Read the model definition and answer for the solid it produces. Units are mm, in the model's axes. Coordinates: 2 decimals unless noted, no trailing zeros. Order: outer loops, then holes, each group sorted by start corner. A loop starts at its lowest first (then second) coordinate and runs counter-clockwise, first axis right, second up.
```python
from build123d import *

# Parameters (mm, degrees)
SKETCH1_W           = 500
SKETCH1_H           = 500
BOSS_EXTRUDE1_DEPTH = 6.35
SKETCH2_R           = 84
CUT_EXTRUDE1_DEPTH  = 6.35
CUT_EXTRUDE3_DEPTH  = 6.35
FILLET1_R           = 15


with BuildPart() as part:
    # Sketch1 → Boss-Extrude1 (new body)
    with BuildSketch(Plane(origin=(0, 0, 0), x_dir=(1, 0, 0), z_dir=(0, 1, 0))):
        with Locations((48.037604912, -85.456276451)):
            Rectangle(SKETCH1_W, SKETCH1_H)
    extrude(amount=BOSS_EXTRUDE1_DEPTH)

    # Sketch2 → Cut-Extrude1 (cut)
    with BuildSketch(Plane(origin=(0, 6.35, 0), x_dir=(1, 0, 0), z_dir=(0, 1, 0))):
        with Locations((48.037604912, -85.456276451)):
            Circle(SKETCH2_R)
    extrude(amount=-CUT_EXTRUDE1_DEPTH, mode=Mode.SUBTRACT)

    # Sketch3 → Cut-Extrude3 (cut)
    with BuildSketch(Plane(origin=(0, 6.35, 0), x_dir=(1, 0, 0), z_dir=(0, 1, 0))):
        Polygon((216.329018834, 78.592496784), (103.191933845, -34.544588206), (98.949293158, -30.301947519), (212.086378147, 82.835137471), align=None)
        Polygon((-120.25380901, 78.592496784), (-116.011168323, 82.835137471), (-2.874083333, -30.301947519), (-7.11672402, -34.544588206), align=None)
        Polygon((212.086378147, -253.747690374), (98.949293158, -140.610605384), (103.191933845, -136.367964697), (216.329018835, -249.505049687), align=None)
        Polygon((-120.25380901, -249.505049687), (-7.11672402, -136.367964697), (-2.874083333, -140.610605384), (-116.011168323, -253.747690374), align=None)
    extrude(amount=-CUT_EXTRUDE3_DEPTH, mode=Mode.SUBTRACT)

    # Fillet1
    fillet1_edges = [part.edges().sort_by_distance(p)[0] for p in [
        (105.275361381, 3.175, 23.975879296),
        (109.518002068, 3.175, 28.218519983),
        (109.518002068, 3.175, 142.69403292),
        (105.275361381, 3.175, 146.936673607),
        (-13.442792244, 3.175, 142.69403292),
        (-9.200151557, 3.175, 146.936673607),
        (-13.442792244, 3.175, 28.218519983),
        (-9.200151557, 3.175, 23.975879296),
    ]]
    fillet(fillet1_edges, radius=FILLET1_R)


solid = part.part
```
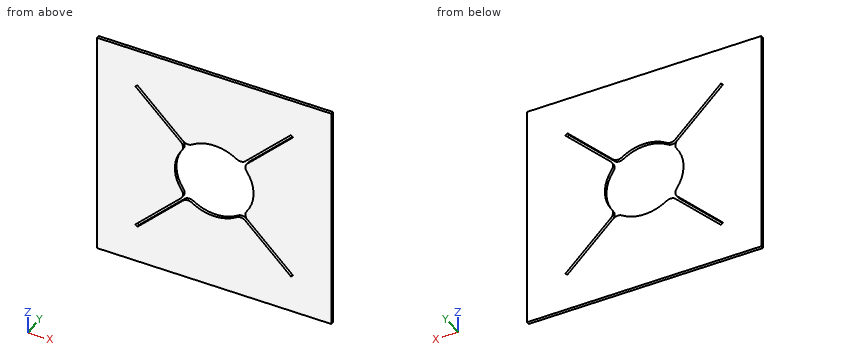
1) A cutting plane is placed at B-B, the plane y = 4.5. Determine the outline of the cut face in (x, z), and give its area (3 significant figures).
A:
outline: (-201.96, -164.54) - (298.04, -164.54) - (298.04, 335.46) - (-201.96, 335.46) - close; hole (-120.25, -78.59) - (-116.01, -82.84) - (-18.68, 14.5) arc R15 cw to (0.43, 16.25) arc R84 ccw to (95.65, 16.25) arc R15 cw to (114.75, 14.5) - (212.09, -82.84) - (216.33, -78.59) - (119, 18.74) arc R15 cw to (117.24, 37.85) arc R84 ccw to (117.24, 133.06) arc R15 cw to (119, 152.17) - (216.33, 249.51) - (212.09, 253.75) - (114.75, 156.41) arc R15 cw to (95.65, 154.66) arc R84 ccw to (0.43, 154.66) arc R15 cw to (-18.68, 156.41) - (-116.01, 253.75) - (-120.25, 249.51) - (-22.92, 152.17) arc R15 cw to (-21.17, 133.06) arc R84 ccw to (-21.17, 37.85) arc R15 cw to (-22.92, 18.74) - close
area: 224,000 mm2
2) A cutting plane is placed at A-A, the plane x = -87. Determine the outline of the cut face in (y, z).
A:
outline: (0, -164.54) - (6.35, -164.54) - (6.35, -53.82) - (0, -53.82) - close; (0, -45.34) - (6.35, -45.34) - (6.35, 216.25) - (0, 216.25) - close; (0, 224.74) - (6.35, 224.74) - (6.35, 335.46) - (0, 335.46) - close
3) A cutting plane is placed at C-C, the plane z = 202.5. Determine the outline of the cut face in (x, y).
A:
outline: (-201.96, 0) - (-73.25, 0) - (-73.25, 6.35) - (-201.96, 6.35) - close; (-64.76, 0) - (160.84, 0) - (160.84, 6.35) - (-64.76, 6.35) - close; (169.32, 0) - (298.04, 0) - (298.04, 6.35) - (169.32, 6.35) - close
4) Straight lines are drawn through the part: line 1 (Z direction, x = -7, y = 4); line 2 (X direction, y = 3, z = -58); line 3 (X direction, y = 5, z = -50). For each, find the intervals that lie inside material, in ascending order.
A:
line 1: z = -164.54 to 18.85, 152.06 to 335.46
line 2: x = -201.96 to -99.66, -91.18 to 187.25, 195.74 to 298.04
line 3: x = -201.96 to -91.66, -83.18 to 179.25, 187.74 to 298.04
